```python
from build123d import *

# Parameters (mm, degrees)
F0_W     = 598
F0_H     = 356
F0_R     = 2
F0_R_2   = 2.053233
F1_DEPTH = 0.5
F2_R     = 5.5
F3_DEPTH = 0.5


with BuildPart() as f1:
    # F0 (on Front) → F1 (new body)
    with BuildSketch(Plane.XZ):
        Rectangle(F0_W, F0_H)
        with Locations((-37.5, -49)):
            Circle(F0_R, mode=Mode.SUBTRACT)
        with Locations((37.5, -49)):
            Circle(F0_R, mode=Mode.SUBTRACT)
        with Locations((-37.5, 26)):
            Circle(F0_R, mode=Mode.SUBTRACT)
        Circle(F0_R_2, mode=Mode.SUBTRACT)
        with Locations((37.5, 26)):
            Circle(F0_R, mode=Mode.SUBTRACT)
    extrude(amount=F1_DEPTH)

    # F2 (on face) → F3 (cut, through all)
    with BuildSketch(Plane.XZ.offset(0.5)):
        with Locations((0, 152.6)):
            Circle(F2_R)
        with Locations((68, 152.6)):
            Circle(F2_R)
        with Locations((136, 152.6)):
            Circle(F2_R)
        with Locations((204, 152.6)):
            Circle(F2_R)
        with Locations((272, 152.6)):
            Circle(F2_R)
        with Locations((272, 91.6)):
            Circle(F2_R)
        with Locations((273.05, 30.48)):
            Circle(F2_R)
        with Locations((273.05, -30.48)):
            Circle(F2_R)
        with Locations((272, -91.6)):
            Circle(F2_R)
        with Locations((-136, 152.6)):
            Circle(F2_R)
        with Locations((-68, 152.6)):
            Circle(F2_R)
        with Locations((-204, 152.6)):
            Circle(F2_R)
        with Locations((-272, 152.6)):
            Circle(F2_R)
        with Locations((-272, -91.6)):
            Circle(F2_R)
        with Locations((-272, -152.6)):
            Circle(F2_R)
        with Locations((-204, -152.6)):
            Circle(F2_R)
        with Locations((272, -152.6)):
            Circle(F2_R)
        with Locations((-272, 91.6)):
            Circle(F2_R)
        with Locations((-68, -152.6)):
            Circle(F2_R)
        with Locations((-273.05, 30.48)):
            Circle(F2_R)
        with Locations((136, -152.6)):
            Circle(F2_R)
        with Locations((68, -152.6)):
            Circle(F2_R)
        with Locations((0, -152.6)):
            Circle(F2_R)
        with Locations((-136, -152.6)):
            Circle(F2_R)
        with Locations((-273.05, -30.48)):
            Circle(F2_R)
        with Locations((204, -152.6)):
            Circle(F2_R)
    extrude(amount=-F3_DEPTH, mode=Mode.SUBTRACT)


solid = f1.part
```
Model file for the job. Use its own axes, mm. Coordinates: 2 decimals unless noted, no trailing zeros. Return JSON: item names as keys, results as strings.
Item 1: Wall check: line 1 along Z through (x, y) = (-136, -0.2); line 2 along X through (y, z) = (-0.3, -29.5); line 3 along Z through (x, y) = (0, -0.2). Give the ranges that are in metal, low to high. Write a range as from..to.
Model answer:
{"line 1": "z = -178..-158.1, -147.1..147.1, 158.1..178", "line 2": "x = -299..-278.46, -267.64..267.64, 278.46..299", "line 3": "z = -178..-158.1, -147.1..-2.05, 2.05..147.1, 158.1..178"}
Item 2: Pin check, flat tips, straight feed: P1, Ø9, axis at x = -136, z = -152.6, coming from the -Y side; P2, Ø1.5, axis at x = 132.5, z = 2, coming from the +Y side. Stop position of each tip, or through.
Model answer:
{"P1": "passes through", "P2": "stops at y = 0"}
Item 3: Mould opens along X. For faces 1 (the face through (-4, -0.5, 2)), 2 (the face through (63.95, -0.25, -148.88)) say: pulls with the +X half, pulls with the -X half, needs draft (parallel to the pull), parting line crosses it, or undercut.
Model answer:
{"face 1": "needs draft", "face 2": "undercut"}
